Geometry check sheet. Reference: the model listing, model coordinates, mm. A direction names the side the tool comes from. Give positions to 0.01 mm unless a question says otherwise; leave off trailing zeros. Write each loop counter-clockwise with the first axis right and the second up, starting at its lowest first coordinate (ties: lowest second). Pieces come first, ordered by that corner, then holes. Notation, with made-up numbers: (81, 45.5) -> (91, 45.5) arc R22 cw to (91, 54.5) -> close; hole circle Ø3 at (-6, -18.5). An arc over 180 degrees is marked (long way). Write item = value, one per line. Start each with the question number.
1. Cross-section at C-C, the plane x = -4.5. Record the cut outline in (y, z).
2. Set-up check for faces 1 (the flat face through (29, -60, 21.512)), 2 (the flat face through (46.099, -60, 4)), 3 (the flat face through (37, 45, 0)), 4 (the cylindrical face through (14.32, -61, -11.61)), 5 (the cylindrical face through (44.67, -61, 20.01)): record each of +Z, -Z, +X, -X, +Y, -Y from which the full face is reachable in a straight line by a thin tool's end or side.
3. Cross-section at B-B, the plane z = -26.5. Record the cut outline in (x, y).
4. Thickness scan on line 1 along Y through (x, z) = (25, 32.5); line 2 along Y through (x, z) = (15.5, 18.5); line 3 along X through (y, z) = (65, -8.5). Record the ranges inside material, lowest first.
5. Cross-section at A-A, the plane y = -42. Record the cut outline in (x, z), plus the area to 3 significant figures.
6. Cross-section at D-D, the plane y = 65. Record the cut outline in (x, z).
7. Depth check by flat-ended pin: P1, Ø24.5, axis at x = 32.5, y = 64.5, coming from the +Z side; P2, Ø7.5, axis at y = -65.5, z = 5, coming from the +X side; P3, Ø8, axis at x = 21.5, z = 19.5, coming from the +Y side. Enter the tip coordinate at first touch or a pass-through.
```python
from build123d import *

# Parameters (mm, degrees)
F0_W     = 73.031641
F0_H     = 84.304981
F1_DEPTH = 25
F2_W     = 33.280658
F2_H     = 34.5481
F3_DEPTH = 71
F4_R     = 5
F5_R     = 5.836703
F6_DEPTH = 49.1
F7_W     = 22.180748
F7_H     = 17.729454
F8_DEPTH = 90.629987
F9_R     = 3


with BuildPart() as f1:
    # F0 (on Front) → F1 (new body)
    with BuildSketch(Plane.XZ):
        with Locations((23.036827, 2.042271)):
            Rectangle(F0_W, F0_H)
    extrude(amount=F1_DEPTH)

    # F2 (on face) → F3 (join)
    with BuildSketch(Plane.XZ.offset(25)):
        with Locations((29.459043, 4.238339)):
            Rectangle(F2_W, F2_H)
    extrude(amount=F3_DEPTH)

    # F4
    f4_edges = [f1.edges().sort_by_distance(p)[0] for p in [
        (46.099372, -60.5, -13.035711),
        (46.099372, -60.5, 21.512389),
        (12.818714, -60.5, 21.512389),
        (12.818714, -60.5, -13.035711),
    ]]
    fillet(f4_edges, radius=F4_R)

    # F5 (on face) → F6 (join)
    with BuildSketch(Plane.XZ.offset(96)):
        with Locations((29.61137, 8.004888)):
            Circle(F5_R)
    extrude(amount=F6_DEPTH)

    # F7 (on face) → F8 (join)
    with BuildSketch(Plane(origin=(0, 0, 0), x_dir=(-1, 0, 0), z_dir=(0, 1, 0))):
        with Locations((-37.29094, -8.864727)):
            Rectangle(F7_W, F7_H)
    extrude(amount=F8_DEPTH)

    # F9
    f9_edges = [f1.edges().sort_by_distance(p)[0] for p in [
        (26.200566, 45.314994, -17.729454),
        (48.381314, 45.314994, -17.729454),
    ]]
    fillet(f9_edges, radius=F9_R)


solid = f1.part
```
Answers:
q1.outline = (-25, -40.11) -> (0, -40.11) -> (0, 44.19) -> (-25, 44.19) -> close
q2.face_1 = +Z, +X, -X, -Y
q2.face_2 = +Z, -Z, +X, -Y
q2.face_3 = +Z, +X, -X, +Y
q2.face_4 = -Z, -X, -Y
q2.face_5 = +Z, +X, -Y
q3.outline = (-13.48, -25) -> (59.55, -25) -> (59.55, 0) -> (-13.48, 0) -> close
q4.line_1 = -25 to 0
q4.line_2 = -96 to 0
q4.line_3 = 26.2 to 48.38
q5.outline = (12.82, -8.04) arc R5 ccw to (17.82, -13.04) -> (41.1, -13.04) arc R5 ccw to (46.1, -8.04) -> (46.1, 16.51) arc R5 ccw to (41.1, 21.51) -> (17.82, 21.51) arc R5 ccw to (12.82, 16.51) -> close
q5.area = 1,130 mm^2
q6.outline = (26.2, -14.73) arc R3 ccw to (29.2, -17.73) -> (45.38, -17.73) arc R3 ccw to (48.38, -14.73) -> (48.38, 0) -> (26.2, 0) -> close
q7.P1 = 0
q7.P2 = 46.1
q7.P3 = 0
